from build123d import *

# Parameters (mm, degrees)
F1_W     = 51.249427
F1_H     = 10.54919
F2_DEPTH = 25.4
F0_W     = 51.912584
F0_H     = 98.145824
F3_DEPTH = 6.35
F4_R     = 3.175
F4_R_2   = 5.08
F5_DEPTH = 25.4


with BuildPart() as f2:
    # F1 (on Top) → F2 (new body)
    with BuildSketch(Plane.XY):
        with Locations((9.770837, -35.216718)):
            Rectangle(F1_W, F1_H)
    extrude(amount=F2_DEPTH)

    # F0 (on Top) → F3 (join)
    with BuildSketch(Plane.XY):
        with Locations((9.720873, 8.55908)):
            Rectangle(F0_W, F0_H)
    extrude(amount=-F3_DEPTH)

    # F4 (on face) → F5 (cut)
    with BuildSketch(Plane.XY):
        with Locations((-6.719237, 45.145492)):
            Circle(F4_R)
        with Locations((-6.752275, 19.745523)):
            Circle(F4_R)
        with Locations((-6.710419, -6.288796)):
            Circle(F4_R)
        with Locations((22.977165, 44.904832)):
            Circle(F4_R_2)
    extrude(amount=-F5_DEPTH, mode=Mode.SUBTRACT)


solid = f2.part
Build history of the part. All positions in model axes, mm. A direction names the side the tool comes from. Round coordinates to 2 decimals unless told otherwise and drop trailing zeros. Write each loop counter-clockwise with the first axis right and the second up, starting at its lowest first coordinate (ties: lowest second). Pieces come first, ordered by that corner, then holes. Notation, with made-up numbers: M 40.25,89 L 80.25,89 A9 ccw 80.25,103 Z; hole C 29.25,86.25 d6. An arc over 180 degrees is marked long. Answer as a JSON object with one key per item and string values. Group by question number.
(1) Cut at A-A (x = -7). Give the number of separate pieces and of enclosed holes in the cut face, and give its area (3 significant figures).
(2) Cut at D-D (z = 16). Give the cut face in (x, y).
(3) Mould opens along Y. For faces 4 (the flat face through (35.677, 8, -3)), 5 (the flat face through (9, 57.632, -3)), 6 (the cylindrical face through (-7.12, -3.14, -3.13)) say: pulls with the +Y half, pulls with the -Y half, needs draft (parallel to the pull), parting line crosses it, or undercut.
(4) Flat gauge pins, fed straight in: pin 1 (5 mm diameter, centred on x = -4, z = 19, fed in from +Y); pin 2 (10 mm diameter, centred on x = -6.71, y = -6.29, fed in from -Z); pin 3 (3 mm diameter, centred on y = -33.5, z = 10.5, fed in from +X); pin 4 (11.5 mm diameter, centred on x = 22.98, y = 44.9, fed in from +Z). Where does each tip first touch, or does it go through?
(5) Which spindle directions (+Z, -Z, +X, -X, +Y, -Y) get a long thin tool onto all of the face, cutting with end or side? Do faces 1 (the flat face through (35.396, -35, 13)), 2 (the flat face through (9, -29.942, 13)), 3 (the flat face through (-15.854, -35, 13)). Say none if no direction does.
(6) Drill centre lines: L1, parallel to Y at x = 9, z = 7.5; L2, parallel to Z at x = -4.5, y = 2; L3, parallel to X at y = -34.5, z = 23.5. Where is each one in solid material? Low to high.
Responses:
{
 "1": {"separate pieces": "4", "enclosed holes": "0", "area": "771 mm2"},
 "2": {"outline": "M -15.85,-40.49 L 35.4,-40.49 L 35.4,-29.94 L -15.85,-29.94 Z"},
 "3": {"face 4": "needs draft", "face 5": "pulls with the +Y half", "face 6": "undercut"},
 "4": {"pin 1": "stops at y = -29.94", "pin 2": "stops at z = -6.35", "pin 3": "stops at x = 35.4", "pin 4": "stops at z = 0"},
 "5": {"face 1": "+Z, +X, +Y, -Y", "face 2": "+Z, +X, -X, +Y", "face 3": "+Z, -X, +Y, -Y"},
 "6": {"L1": "y = -40.49 to -29.94", "L2": "z = -6.35 to 0", "L3": "x = -15.85 to 35.4"}
}
